from build123d import *

# Parameters (mm, degrees)
SKETCH1_R           = 82.55
SKETCH1_R_2         = 18.415
BOSS_EXTRUDE3_DEPTH = 25.4
SKETCH1_7_W         = 42.799
SKETCH1_7_H         = 42.799
CUT_EXTRUDE2_DEPTH  = 20.5
SKETCH3_W           = 25.4
SKETCH3_H           = 15.24
CUT_EXTRUDE3_DEPTH  = 120.474537036
SKETCH1_8_R         = 2.75
CUT_EXTRUDE4_DEPTH  = 6
CUT_EXTRUDE5_START  = 19.4
SKETCH1_10_R        = 2.75
CUT_EXTRUDE5_DEPTH  = 6


with BuildPart() as part:
    # Sketch1 → Boss-Extrude3 (new body)
    with BuildSketch(Plane(origin=(0, 0, 0), x_dir=(1, 0, 0), z_dir=(0, 1, 0))):
        with Locations(Location((0, 0, 0), (0, 0, 270))):
            Circle(SKETCH1_R)
        with Locations(Location((0, 57.785, 0), (0, 0, 270))):
            Circle(SKETCH1_R_2, mode=Mode.SUBTRACT)
    extrude(amount=BOSS_EXTRUDE3_DEPTH)

    # Sketch1_7 → Cut-Extrude2 (cut)
    with BuildSketch(Plane(origin=(0, 0, 0), x_dir=(1, 0, 0), z_dir=(0, 1, 0))):
        Rectangle(SKETCH1_7_W, SKETCH1_7_H)
    extrude(amount=CUT_EXTRUDE2_DEPTH, mode=Mode.SUBTRACT)

    # Sketch3 → Cut-Extrude3 (cut, through all)
    with BuildSketch(Plane.XZ):
        with Locations((0, 29.0195)):
            Rectangle(SKETCH3_W, SKETCH3_H)
    extrude(amount=-CUT_EXTRUDE3_DEPTH, mode=Mode.SUBTRACT)

    # Sketch1_8 → Cut-Extrude4 (cut)
    with BuildSketch(Plane(origin=(0, 0, 0), x_dir=(1, 0, 0), z_dir=(0, 1, 0))):
        with Locations(Location((-49.53, -49.53, 0), (0, 0, 270))):
            Circle(SKETCH1_8_R)
        with Locations(Location((49.53, -49.53, 0), (0, 0, 270))):
            Circle(SKETCH1_8_R)
        with Locations(Location((-49.53, 49.53, 0), (0, 0, 270))):
            Circle(SKETCH1_8_R)
        with Locations(Location((49.53, 49.53, 0), (0, 0, 270))):
            Circle(SKETCH1_8_R)
    extrude(amount=CUT_EXTRUDE4_DEPTH, mode=Mode.SUBTRACT)

    # Sketch1_10 → Cut-Extrude5 (cut)
    with BuildSketch(Plane(origin=(0, 0, 0), x_dir=(1, 0, 0), z_dir=(0, 1, 0)).offset(CUT_EXTRUDE5_START)):
        with Locations(Location((-49.53, 49.53, 0), (0, 0, 270))):
            Circle(SKETCH1_10_R)
        with Locations(Location((49.53, 49.53, 0), (0, 0, 270))):
            Circle(SKETCH1_10_R)
        with Locations(Location((-49.53, -49.53, 0), (0, 0, 270))):
            Circle(SKETCH1_10_R)
        with Locations(Location((49.53, -49.53, 0), (0, 0, 270))):
            Circle(SKETCH1_10_R)
    extrude(amount=CUT_EXTRUDE5_DEPTH, mode=Mode.SUBTRACT)


solid = part.part
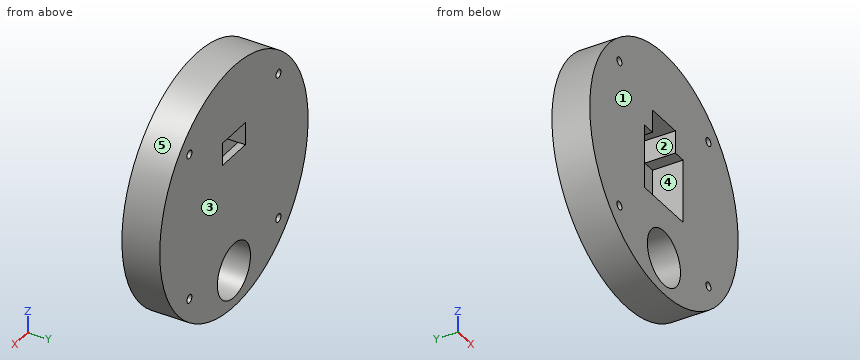
Source: CAD feature listing. Evaluate the final solid. Frame: model axes, mm. Face numbers are marked on the shaded views. A direction names the side the tool comes from. Coordinates: 2 decimals unless noted, no trailing zeros. Loops run counter-clockwise (first coordinate to the right, second up) from the corner with the lowest first, then second, coordinate; pieces in that order, holes last. Notation, with made-up numbers: M -12.75,38 L 2.25,38 A23 ccw 2.25,63 Z; hole C 87.25,27 d3. An arc over 180 degrees is marked long. Answer in a Markdown table with one row per item.
Q1. Draft query along Z for the marked faces 3, 4 and 5. Return one class per face: pulls with the +Z half, pulls with the -Z half, needs draft (parallel to the pull), parting line crosses it, or undercut.
Answers below:
| item | result |
|---|---|
| face 3 | needs draft |
| face 4 | undercut |
| face 5 | parting line crosses it |
Q2. Section A-A on y = 2.5. State how many separate pieces and enclosed holes the cut face has, plus the area to 3 significant figures.
Answers below:
| item | result |
|---|---|
| separate pieces | 1 |
| enclosed holes | 6 |
| area | 18,000 mm^2 |
Q3. Ray query, probe 1 along X at (y, z) = (20.7, -49.53); probe 2 along X at (y, z) = (11.5, 0); probe 3 along X at (y, z) = (3.8, 49.53). Return the intervals inside material, ascending. Write a range as from..to.
Answers below:
| item | result |
|---|---|
| probe 1 | x = -66.04..-52.28, -46.78..-16.46, 16.46..46.78, 52.28..66.04 |
| probe 2 | x = -82.55..-21.4, 21.4..82.55 |
| probe 3 | x = -66.04..-52.28, -46.78..46.78, 52.28..66.04 |
Q4. Section C-C on z = 28. Return the cut outline in (x, y), plus the area to 3 significant figures.
Answers below:
| item | result |
|---|---|
| outline | M -77.66,0 L -12.7,0 L -12.7,25.4 L -77.66,25.4 Z; M 12.7,0 L 77.66,0 L 77.66,25.4 L 12.7,25.4 Z |
| area | 3,300 mm^2 |
Q5. First-contact query: pin 1 (4.5 mm diameter, centred on x = -49.53, z = -49.53, fed in from +Y); pin 2 (7.5 mm diameter, centred on y = 16, z = 31, fed in from -X); pin 3 (4 mm diameter, centred on x = 2.5, y = 23, fed in from +Z). Flat tips, straight axial feed; report the tip coordinate or a pass-through.
Answers below:
| item | result |
|---|---|
| pin 1 | stops at y = 19.4 |
| pin 2 | stops at x = -77.92 |
| pin 3 | stops at z = 82.55 |
Q6. Set-up query: the marked faces 1 and 2. Return all of +Z, -Z, +X, -X, +Y, -Y with unobstructed straight access to the full face (end or side cutting, diameter ignored); none if empty.
Answers below:
| item | result |
|---|---|
| face 1 | +Z, -Z, +X, -X, -Y |
| face 2 | +Y, -Y |
Q7. Section B-B on x = 0. Return the cut outline in (y, z).
Answers below:
| item | result |
|---|---|
| outline | M 0,-82.55 L 25.4,-82.55 L 25.4,-76.2 L 0,-76.2 Z; M 0,-39.37 L 25.4,-39.37 L 25.4,21.4 L 20.5,21.4 L 20.5,-21.4 L 0,-21.4 Z; M 0,36.64 L 25.4,36.64 L 25.4,82.55 L 0,82.55 Z |
